Here's the drawing with two shaded views (mm, measured from the low corner). I have some questions. A direction names the side the tool comes from. Give positions to 0.01 mm unless a question says otherwise; leave off trailing zeros. Loops run counter-clockwise (first coordinate to the right, second up) from the corner with the lowest first, then second, coordinate; pieces in that order, holes last. Notation, with made-up numbers: M -18,52 L 9,52 A30 cw 9,78 Z; hole C -19.75,25 d3. An arc over 180 degrees is marked long. Answer in a Markdown table with one row per item. Add a question column.
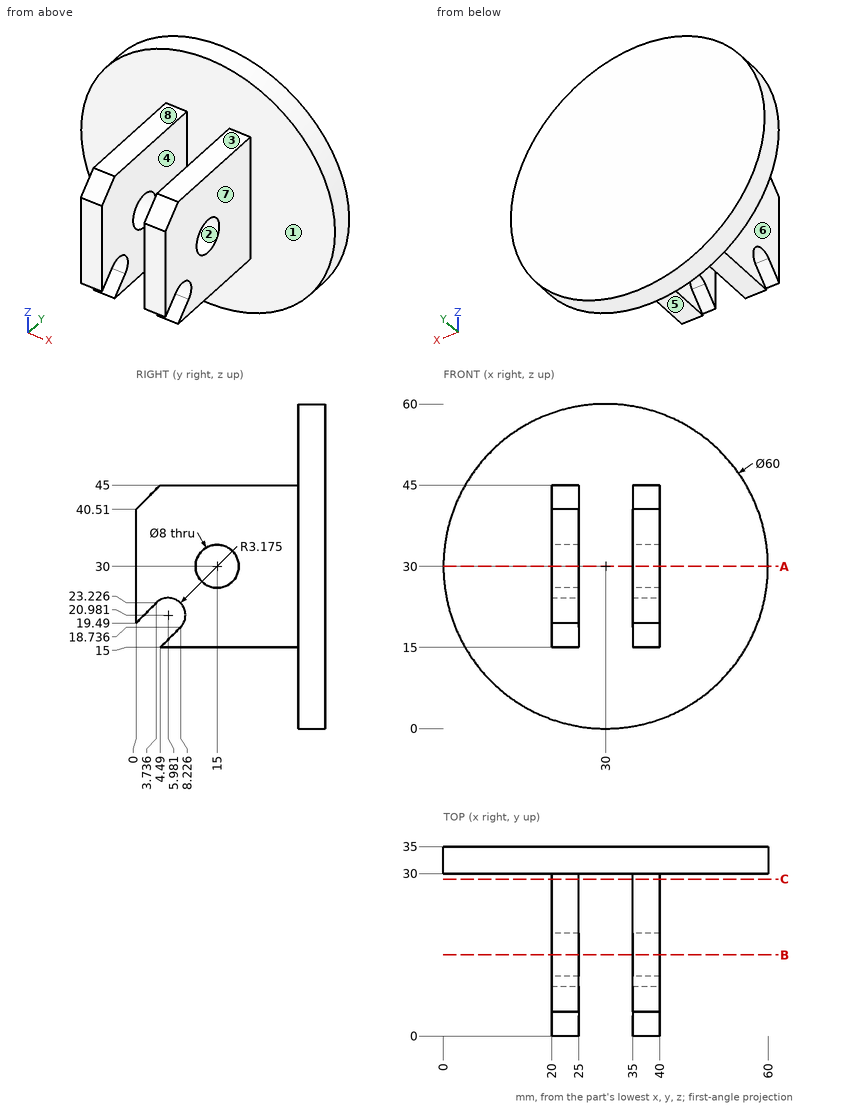
Item 1: Suppose I cut it at C-C (y = 29). List the corners of the cut face in (x, z) for me, then the cut area to 3 significant figures.
Item 2: I need wall thicknesses on L1, parallel to X at y = 25.5, z = 22.5; L2, parallel to Z at x = 38.05, y = 15; L3, parallel to Y at x = 21.65, z = 30. Which ranges of each line are inside material? Lowest first, please.
Item 3: If we mould it in two halves opening along Z, with no side actions, what happens to the marked faces 1, 2 and 3? For each: +Z half, -Z half, draft (parallel to the pull), parting line (faces both ways), or undercut.
Item 4: For the marked faces 4, 5, 6, 7 and 8, which set-ups out of +Z, -Z, +X, -X, +Y, -Y let a thin tool reach every point of the face, with its end or its side?
Item 5: Suppose I cut it at A-A (z = 30). List the corners of the cut face in (x, y) for me.
Item 6: For P1, Ø1.5, axis at x = 21.5, y = 11, coming from the +Z side; P2, Ø10, axis at y = 18, z = 25, coming from the +X side; P3, Ø5, axis at y = 21.5, z = 29.5, coming from the -X side, each with a flat end and sliding along its axis, tell me the tip position at first contact or that it passes through.
Item 7: Suppose I cut it at B-B (y = 15). List the corners of the cut face in (x, z) for me, then the cut area to 3 significant figures.
Values found:
| question | item | result |
|---|---|---|
| 1 | outline | M 20,15 L 25,15 L 25,45 L 20,45 Z; M 35,15 L 40,15 L 40,45 L 35,45 Z |
| 1 | area | 300 mm² |
| 2 | L1 | 20 to 25, 35 to 40 |
| 2 | L2 | 15 to 26, 34 to 45 |
| 2 | L3 | 0 to 11, 19 to 35 |
| 3 | face 1 | draft |
| 3 | face 2 | undercut |
| 3 | face 3 | +Z half |
| 4 | face 4 | +Z, -Z, -Y |
| 4 | face 5 | -Z, +X, -X, -Y |
| 4 | face 6 | +Z, -Z, -X, -Y |
| 4 | face 7 | +Z, -Z, +X, -Y |
| 4 | face 8 | +Z, +X, -X, -Y |
| 5 | outline | M 0,30 L 20,30 L 20,19 L 25,19 L 25,30 L 35,30 L 35,19 L 40,19 L 40,30 L 60,30 L 60,35 L 0,35 Z; M 20,0 L 25,0 L 25,11 L 20,11 Z; M 35,0 L 40,0 L 40,11 L 35,11 Z |
| 6 | P1 | z = 45 |
| 6 | P2 | x = 40 |
| 6 | P3 | x = 20 |
| 7 | outline | M 20,15 L 25,15 L 25,26 L 20,26 Z; M 20,34 L 25,34 L 25,45 L 20,45 Z; M 35,15 L 40,15 L 40,26 L 35,26 Z; M 35,34 L 40,34 L 40,45 L 35,45 Z |
| 7 | area | 220 mm² |
